from build123d import *

# Parameters (mm, degrees)
SKETCH1_W            = 45.3
SKETCH1_H            = 20.05
BOSS_EXTRUDE1_DEPTH  = 3
SKETCH2_R            = 8.5
CUT_EXTRUDE1_DEPTH   = 4
SKETCH3_W            = 8.4
SKETCH3_H            = 4.7
CUT_EXTRUDE2_DEPTH   = 1
SKETCH10_W           = 16.728431373
SKETCH10_H           = 3
BOSS_EXTRUDE8_DEPTH  = 10
SKETCH11_W           = 13.5
SKETCH11_H           = 10
BOSS_EXTRUDE9_DEPTH  = 20
SKETCH12_W           = 13.5
SKETCH12_H           = 2.12
CUT_EXTRUDE3_DEPTH   = 10
SKETCH13_W           = 13.5
SKETCH13_H           = 4
BOSS_EXTRUDE10_DEPTH = 6
SKETCH14_W           = 4
SKETCH14_H           = 3
BOSS_EXTRUDE11_DEPTH = 32
SKETCH15_W           = 32
SKETCH15_H           = 4
BOSS_EXTRUDE12_DEPTH = 3
SKETCH16_W           = 45.5
SKETCH16_H           = 6
BOSS_EXTRUDE13_DEPTH = 33
SKETCH17_W           = 18.3
SKETCH17_H           = 20
CUT_EXTRUDE4_DEPTH   = 7
SKETCH18_R           = 1.5
CUT_EXTRUDE5_DEPTH   = 7
SKETCH20_W           = 10.008836356
SKETCH20_H           = 4.284437553
CUT_EXTRUDE6_DEPTH   = 46.5
SKETCH21_W           = 8.4
SKETCH21_H           = 4.7
CUT_EXTRUDE7_DEPTH   = 3


with BuildPart() as part:
    # Sketch1 → Boss-Extrude1 (new body)
    with BuildSketch(Plane.XY):
        with Locations((22.65, 10.025)):
            Rectangle(SKETCH1_W, SKETCH1_H)
    extrude(amount=BOSS_EXTRUDE1_DEPTH)

    # Sketch2 → Cut-Extrude1 (cut, through all)
    with BuildSketch(Plane.XY.offset(3)):
        with Locations((9.95, 10.025)):
            Circle(SKETCH2_R)
        with Locations((35.35, 10.025)):
            Circle(SKETCH2_R)
        with BuildLine():
            Line((19.45, 19.255641391), (25.85, 19.255641391))
            ThreePointArc((25.85, 19.255641391), (28.155641391, 16.95), (25.85, 14.644358609))
            Line((25.85, 14.644358609), (19.45, 14.644358609))
            ThreePointArc((19.45, 14.644358609), (17.144358609, 16.95), (19.45, 19.255641391))
        make_face()
    extrude(amount=-CUT_EXTRUDE1_DEPTH, mode=Mode.SUBTRACT)

    # Sketch3 → Cut-Extrude2 (cut)
    with BuildSketch(Plane.XY.offset(3)):
        with Locations((22.65, 2.35)):
            Rectangle(SKETCH3_W, SKETCH3_H)
    extrude(amount=-CUT_EXTRUDE2_DEPTH, mode=Mode.SUBTRACT)

    # Sketch10 → Boss-Extrude8 (add)
    with BuildSketch(Plane.XZ):
        with Locations((8.364215686, 1.5)):
            Rectangle(SKETCH10_W, SKETCH10_H)
        with Locations((36.935784314, 1.5)):
            Rectangle(SKETCH10_W, SKETCH10_H)
    extrude(amount=BOSS_EXTRUDE8_DEPTH)

    # Sketch11 → Boss-Extrude9 (add)
    with BuildSketch(Plane.XY.offset(3)):
        with Locations((6.75, -5)):
            Rectangle(SKETCH11_W, SKETCH11_H)
        with Locations((38.55, -5)):
            Rectangle(SKETCH11_W, SKETCH11_H)
    extrude(amount=BOSS_EXTRUDE9_DEPTH)

    # Sketch12 → Cut-Extrude3 (cut)
    with BuildSketch(Plane.XY.offset(23)):
        with Locations((6.75, -4.750002431)):
            Rectangle(SKETCH12_W, SKETCH12_H)
        with Locations((38.55, -4.750002431)):
            Rectangle(SKETCH12_W, SKETCH12_H)
    extrude(amount=-CUT_EXTRUDE3_DEPTH, mode=Mode.SUBTRACT)

    # Sketch13 → Boss-Extrude10 (add)
    with BuildSketch(Plane.XZ.offset(10)):
        with Locations((6.75, 2)):
            Rectangle(SKETCH13_W, SKETCH13_H)
    extrude(amount=BOSS_EXTRUDE10_DEPTH)

    # Sketch14 → Boss-Extrude11 (add)
    with BuildSketch(Plane(origin=(13.5, 0, 0), x_dir=(0, 0, -1), z_dir=(1, 0, 0))):
        with Locations((-2, -14.5)):
            Rectangle(SKETCH14_W, SKETCH14_H)
    extrude(amount=BOSS_EXTRUDE11_DEPTH)

    # Sketch15 → Boss-Extrude12 (add)
    with BuildSketch(Plane(origin=(0, -13, 0), x_dir=(1, 0, 0), z_dir=(0, 1, 0))):
        with Locations((29.5, -2)):
            Rectangle(SKETCH15_W, SKETCH15_H)
    extrude(amount=BOSS_EXTRUDE12_DEPTH)

    # Sketch16 → Boss-Extrude13 (add)
    with BuildSketch(Plane.XY.offset(4)):
        with Locations((22.75, -13)):
            Rectangle(SKETCH16_W, SKETCH16_H)
    extrude(amount=BOSS_EXTRUDE13_DEPTH)

    # Sketch17 → Cut-Extrude4 (cut, through all)
    with BuildSketch(Plane(origin=(0, -10, 0), x_dir=(1, 0, 0), z_dir=(0, 1, 0))):
        with Locations((22.65, -13)):
            Rectangle(SKETCH17_W, SKETCH17_H)
    extrude(amount=-CUT_EXTRUDE4_DEPTH, mode=Mode.SUBTRACT)

    # Sketch18 → Cut-Extrude5 (cut, through all)
    with BuildSketch(Plane(origin=(0, -10, 0), x_dir=(1, 0, 0), z_dir=(0, 1, 0))):
        with Locations((6.75, -30)):
            Circle(SKETCH18_R)
        with Locations((38.648372532, -29.772154482)):
            Circle(SKETCH18_R)
    extrude(amount=-CUT_EXTRUDE5_DEPTH, mode=Mode.SUBTRACT)

    # Sketch20 → Cut-Extrude6 (cut, through all)
    with BuildSketch(Plane.ZY):
        with Locations((17.995581822, -7.952221208)):
            Rectangle(SKETCH20_W, SKETCH20_H)
    extrude(amount=-CUT_EXTRUDE6_DEPTH, mode=Mode.SUBTRACT)

    # Sketch21 → Cut-Extrude7 (cut, through all)
    with BuildSketch(Plane.XY.offset(2)):
        with Locations((22.65, 2.35)):
            Rectangle(SKETCH21_W, SKETCH21_H)
    extrude(amount=-CUT_EXTRUDE7_DEPTH, mode=Mode.SUBTRACT)


solid = part.part
Model file for the job. Use its own axes, mm. A direction names the side the tool comes from. Round coordinates to 2 decimals unless told otherwise and drop trailing zeros. Order: outer loops, then holes, each group sorted by start corner. A loop starts at its lowest first (then second) coordinate and runs counter-clockwise, first axis right, second up.
(1) Band-saw the part on A-A (z = 21.5). List the corners of the cut face in (x, y).
(2) Band-saw the part on C-C (y = 16.95). List the corners of the cut face in (x, z).
(3) 3-axis set-ups, long thin cutter, end or side, ignore diameter. For faces 1 (the face through (7, -5, 13)), 2 (the face through (39, -10.094, 18)), 3 (the face through (31.8, -8, 11)), 4 (the face through (28.572, -5, 1)): which of +Z, -Z, +X, -X, +Y, -Y reach the whole face in a straight line?
(4) Pull direction X, two halves, no side cores. Call faces 5 (the face through (7, 0, 13)), 6 (the face through (26.85, 2, 2)): released by +X, released by -X, zero draft, split by the parting line, or undercut.
(5) Drill centre lines: line 1 (Y direction, x = 9.95, z = 1.4) (3 decimals); line 2 (X direction, y = -12, z = 7.5); line 3 (X direction, y = -6.5, z = 12). Where is each one in solid material? Low to high.
(6) Band-saw the part on B-B (x = 35.35). List the corners of the cut face in (y, z) (3 decimals).
(7) Band-saw the part on D-D (z = 6). List the corners of the cut face in (x, y), then the cut area to 3 significant figures.
(8) Pin check, flat tips, straight feed: pin 1 (2.5 mm diameter, centred on x = 41.5, y = -5, fed in from +Z); pin 2 (12 mm diameter, centred on x = 7.5, y = 2.5, fed in from +Z); pin 3 (8 mm diameter, centred on x = 37, z = 18.5, fed in from +Y). Stop position of each tip, or through.
Verdict:
1. outline: (0, -16) - (13.5, -16) - (13.5, -10.09) - (0, -10.09) - close; (0, -3.69) - (13.5, -3.69) - (13.5, 0) - (0, 0) - close; (31.8, -16) - (45.5, -16) - (45.5, -10.09) - (31.8, -10.09) - close; (31.8, -3.69) - (45.3, -3.69) - (45.3, 0) - (31.8, 0) - close
2. outline: (0, 0) - (5.02, 0) - (5.02, 3) - (0, 3) - close; (14.88, 0) - (17.14, 0) - (17.14, 3) - (14.88, 3) - close; (28.16, 0) - (30.42, 0) - (30.42, 3) - (28.16, 3) - close; (40.28, 0) - (45.3, 0) - (45.3, 3) - (40.28, 3) - close
3. face 1: +Z, +X, -X
3. face 2: +X, -X
3. face 3: +Y, -Y
3. face 4: +Z, -Z
4. face 5: zero draft
4. face 6: undercut
5. line 1: y = -16 to 1.525, 18.525 to 20.05
5. line 2: x = 0 to 13.5, 31.8 to 45.5
5. line 3: x = 0 to 13.5, 31.8 to 45.3
6. outline: (-16, 0) - (1.525, 0) - (1.525, 3) - (0, 3) - (0, 23) - (-3.69, 23) - (-3.69, 13) - (-5.81, 13) - (-5.81, 12.991) - (-10.094, 12.991) - (-10.094, 23) - (-10, 23) - (-10, 37) - (-16, 37) - close; (18.525, 0) - (20.05, 0) - (20.05, 3) - (18.525, 3) - close
7. outline: (0, -16) - (13.5, -16) - (13.5, 0) - (0, 0) - close; (31.8, -16) - (45.5, -16) - (45.5, -10) - (45.3, -10) - (45.3, 0) - (31.8, 0) - close
7. area: 433 mm2
8. pin 1: stops at z = 13
8. pin 2: stops at z = 23
8. pin 3: stops at y = 0
